Build history of the part. All positions in model axes, mm. A direction names the side the tool comes from. Give positions to 0.01 mm unless a question says otherwise; leave off trailing zeros. Loops run counter-clockwise (first coordinate to the right, second up) from the corner with the lowest first, then second, coordinate; pieces in that order, holes last. Notation, with made-up numbers: (50.5, -3.75) -> (92.5, -3.75) arc R25 cw to (92.5, 13.25) -> close; hole circle Ø10 at (-34.5, 74.5). An arc over 180 degrees is marked (long way). Answer as a JSON object with one key per item and string values. Group by question number.
Q1. Band-saw the part on C-C, the plane z = 3.5. Write the cut outline in (x, y).
Q2. Drop flat-ended pins along their axis: pin 1 (2 mm diameter, centred on x = 16.5, z = -0.5, fed in from -Y); pin 2 (4 mm diameter, centred on x = 11, y = -5.5, fed in from -Z); pin 3 (4.5 mm diameter, centred on y = -8.5, z = 1, fed in from +X). Give the stop position or say it passes through.
Q3. Wall check: probe 1 along Z at (x, y) = (20, -2.1); probe 2 along Z at (x, y) = (15.25, -1); probe 3 along Y at (x, z) = (-0.25, 3.5). Give the ranges that are in metal, low to high. Write a range as from..to.
Q4. Band-saw the part on A-A, the plane x = 0. Write the cut outline in (y, z).
Q5. Tool access for faces 4 (the flat face through (2.908, -3.49, 12.865)), 5 (the flat face through (16, -4.9, 0)), 6 (the flat face through (16, -2, 2)), 7 (the flat face through (-2.776, -3.49, 12.195)), 8 (the flat face through (13, -1, -2)): list every direction of +Z, -Z, +X, -X, +Y, -Y with a clear straight run to the whole face (end or side of a thin tool).
Q6. Band-saw the part on B-B, the plane y = -4.5. Count the separate pieces of the cut face and the enclosed holes in it, plus the area to 3 significant figures.
Q7. Two-plate mould, pull along Z, no slides. Class faces 1 (the flat face through (1, -2.4, 3)), 2 (the flat face through (11.832, -5, 0)), 3 (the flat face through (6.16, -2.07, 11.68)): pulls with the +Z half, pulls with the -Z half, needs draft (parallel to the pull), parting line crosses it, or undercut.
Q8. Band-saw the part on D-D, the plane x = 17.25. Write the cut outline in (y, z).
from build123d import *

# Parameters (mm, degrees)
F0_W      = 1.0130730125
F0_H      = 4
F1_DEPTH  = 9.8
F0_R      = 3
F2_DEPTH  = 3
F0_W_2    = 2
F0_R_2    = 1.5
F3_DEPTH  = 4.9
F4_R      = 3
F5_DEPTH  = 9.8
F6_DEPTH  = 2.4
F7_R      = 2.5
F8_DEPTH  = 1.5
F9_SIZE   = 1.49999
F10_DEPTH = 3


# Not quite as in the source:
# - a fillet or chamfer is up to 0.001 mm smaller than in the source, because OpenCascade refuses the exact size
# - a feature names something its author has since deleted; it is built from what else it names


with BuildPart() as f1:
    # F0 (on Front) → F1 (new body)
    with BuildSketch(Plane.XZ):
        with BuildLine():
            ThreePointArc((-2.6630696544, 11.7007717701), (6.6741513084, 9.9727480823), (11.8321595662, 2))
            Line((11.8321595662, 2), (12.8452325787, 2))
            ThreePointArc((12.8452325787, 2), (11.9653059951, 5.0824651934), (10.3578419044, 7.8558965804))
            ThreePointArc((10.3578419044, 7.8558965804), (6.8410523386, 11.0544110156), (2.4094924969, 12.7747542406))
            ThreePointArc((2.4094924969, 12.7747542406), (-0.2428398127, 12.99773168), (-2.8849921256, 12.6758360843))
            Line((-2.8849921256, 12.6758360843), (-2.6630696544, 11.7007717701))
        make_face()
        with Locations((12.3386960724, 0)):
            Rectangle(F0_W, F0_H)
        with BuildLine():
            ThreePointArc((2.4094924969, 12.7747542406), (6.8410523386, 11.0544110156), (10.3578419044, 7.8558965804))
            Line((10.3578419044, 7.8558965804), (8.8443472742, 10.4461347942))
            Line((8.8443472742, 10.4461347942), (3.3933836255, 12.9535229374))
            Line((3.3933836255, 12.9535229374), (2.4094924969, 12.7747542406))
        make_face()
    extrude(amount=F1_DEPTH)

    # F0 (on Front) → F2 (join)
    with BuildSketch(Plane.XZ):
        with Locations((12.3386960724, 0)):
            Rectangle(F0_W, F0_H)
        with BuildLine():
            Line((11.8321595662, 2), (3.4641016151, 2))
            ThreePointArc((3.4641016151, 2), (3.8637033052, 1.0352761804), (4, 0))
            ThreePointArc((4, 0), (3.8637033052, -1.0352761804), (3.4641016151, -2))
            Line((3.4641016151, -2), (11.8321595662, -2))
            Line((11.8321595662, -2), (11.8321595662, 2))
        make_face()
        with BuildLine():
            ThreePointArc((4, 0), (3.8637033052, 1.0352761804), (3.4641016151, 2))
            ThreePointArc((3.4641016151, 2), (-4, 0), (3.4641016151, -2))
            ThreePointArc((3.4641016151, -2), (3.8637033052, -1.0352761804), (4, 0))
        make_face()
        Circle(F0_R, mode=Mode.SUBTRACT)
        Circle(F0_R)
    extrude(amount=-F2_DEPTH)

    # F0 (on Front) → F3 (join)
    with BuildSketch(Plane.XZ):
        with Locations((13.8452325787, 0)):
            Rectangle(F0_W_2, F0_H)
        with BuildLine():
            Line((20, 2), (14.8452325787, 2))
            Line((14.8452325787, 2), (14.8452325787, -2))
            Line((14.8452325787, -2), (20, -2))
            ThreePointArc((20, -2), (22, 0), (20, 2))
        make_face()
        with Locations((20, 0)):
            Circle(F0_R_2, mode=Mode.SUBTRACT)
    extrude(amount=F3_DEPTH)

    # F4 (on face) → F5 (join)
    with BuildSketch(Plane.XZ):
        Circle(F4_R)
    extrude(amount=F5_DEPTH)

    # F4 (on face) → F6 (join)
    with BuildSketch(Plane.XZ):
        with BuildLine():
            ThreePointArc((3.4641016151, -2), (3.8637033052, -1.0352761804), (4, 0))
            ThreePointArc((4, 0), (3.8637033052, 1.0352761804), (3.4641016151, 2))
            ThreePointArc((3.4641016151, 2), (-4, 0), (3.4641016151, -2))
        make_face()
        Circle(F4_R, mode=Mode.SUBTRACT)
    extrude(amount=F6_DEPTH)

    # F7 (on face) → F8 (join)
    with BuildSketch(Plane(origin=(5.5105226193, 0, 11.9796604147), x_dir=(0.9084939414, 0, -0.4178980239), z_dir=(0.4178980239, 0, 0.9084939414))):
        with Locations((0.6696168272, -4.9)):
            Circle(F7_R)
    extrude(amount=F8_DEPTH)

    # F9 (size 1.5 in the source; OpenCascade refuses exactly that, so slightly less here)
    f9_edges = [f1.edges().sort_by_distance(p)[0] for p in [
        (4.474478, -4.9, 14.107315),
    ]]
    chamfer(f9_edges, length=F9_SIZE)

    # F10 (add): a face of the model
    f10_faces = [f1.faces().sort_by_distance(p)[0] for p in [
        (-0.2392542287, 0, 12.8058172707),
    ]]
    extrude(f10_faces, amount=F10_DEPTH)


solid = f1.part
Worked answers:
{
 "1": {"outline": "(-1.94, -2.4) -> (1.94, -2.4) -> (1.94, 3) -> (-1.94, 3) -> close; (11.48, -9.8) -> (12.52, -9.8) -> (12.52, 3) -> (11.48, 3) -> close"},
 "2": {"pin 1": "y = -4.9", "pin 2": "z = -2", "pin 3": "x = 12.85"},
 "3": {"probe 1": "-2..-1.5, 1.5..2", "probe 2": "-2..2", "probe 3": "-2.4..3"},
 "4": {"outline": "(-9.8, -3) -> (-2.4, -3) -> (-2.4, -4) -> (3, -4) -> (3, 4) -> (-2.4, 4) -> (-2.4, 3) -> (-9.8, 3) -> close; (-9.8, 12) -> (3, 12) -> (3, 13) -> (-9.8, 13) -> close"},
 "5": {"face 4": "+Z, +Y, -Y", "face 5": "+Z, -Z, +X, -Y", "face 6": "+Z, +X, +Y, -Y", "face 7": "-X, +Y, -Y", "face 8": "-Z, +X, +Y, -Y"},
 "6": {"separate pieces": "2", "enclosed holes": "1", "area": "88.5 mm2"},
 "7": {"face 1": "undercut", "face 2": "needs draft", "face 3": "pulls with the +Z half"},
 "8": {"outline": "(-4.9, -2) -> (0, -2) -> (0, 2) -> (-4.9, 2) -> close"}
}
